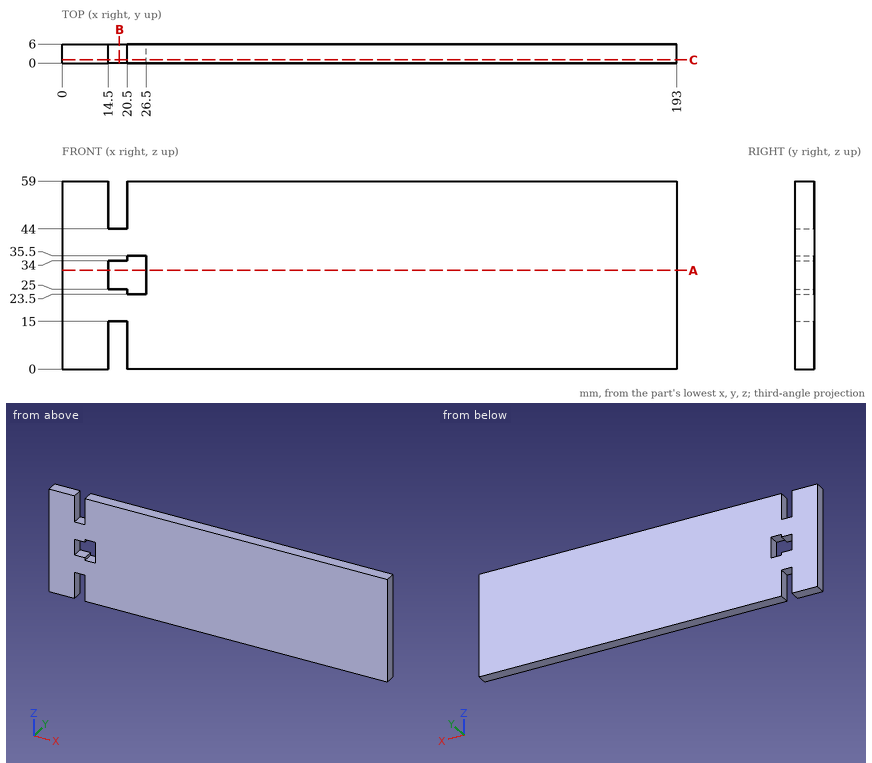
Answer from the drawing. Dimensions are ordinates in mm from the lowest x, y and z of the part. Give positions to 0.01 mm unless a question says otherwise; leave off trailing zeros. Loops run counter-clockwise (first coordinate to the right, second up) from the corner with the lowest first, then second, coordinate; pieces in that order, holes last.
Item 1: Find the intervals of material crossed by line 1 along X through (y, z) = (2.6, 5.5); line 2 along X through (y, z) = (4, 31); line 3 along Z through (x, y) = (17, 5.45), in increasing order.
Item 2: The part is cut by section C-C (y = 1). Write down the section's boundary in (x, z), and give its area (3 significant figures).
Item 3: The part is cut by section B-B (x = 18). Write down the section's boundary in (y, z).
Item 4: This flat-tipped pin is pushed along its axis until it touches: pin 1 Ø1.8 at (x, y) = (17.5, 4.5) entering from +Z. Where does it stop, or does it pass through?
Item 5: The part is cut by section A-A (z = 31). Write down the section's boundary in (x, y), and give its area (3 significant figures).
Taken from the geometry:
1. line 1: x = 0 to 14.5, 20.5 to 193
1. line 2: x = 0 to 14.5, 26.5 to 193
1. line 3: z = 15 to 25, 34 to 44
2. outline: (0, 0) - (14.5, 0) - (14.5, 15) - (20.5, 15) - (20.5, 0) - (193, 0) - (193, 59) - (20.5, 59) - (20.5, 44) - (14.5, 44) - (14.5, 59) - (0, 59) - close; hole (14.5, 25) - (20.5, 25) - (20.5, 23.5) - (26.5, 23.5) - (26.5, 35.5) - (20.5, 35.5) - (20.5, 34) - (14.5, 34) - close
2. area: 11,100 mm2
3. outline: (0, 15) - (6, 15) - (6, 25) - (0, 25) - close; (0, 34) - (6, 34) - (6, 44) - (0, 44) - close
4. pin 1: stops at z = 44
5. outline: (0, 0) - (14.5, 0) - (14.5, 6) - (0, 6) - close; (26.5, 0) - (193, 0) - (193, 6) - (26.5, 6) - close
5. area: 1,090 mm2
